from build123d import *

# Parameters (mm, degrees)
SKETCH1_R                         = 4.9276
BOSS_EXTRUDE1_DEPTH               = 7.9375
SKETCH4_R                         = 4.9276
BOSS_EXTRUDE2_DEPTH               = 3.175
BOSS_EXTRUDE2_TAPER               = 45
F_1_4_20_TAPPED_HOLE1_D           = 5.1054
F_1_4_20_TAPPED_HOLE1_DEPTH       = 16.51
F_1_4_20_TAPPED_HOLE1_CSINK_D     = 8.9154
F_1_4_20_TAPPED_HOLE1_CSINK_ANGLE = 90
F_1_4_20_TAPPED_HOLE1_TIP         = 1.533816902


with BuildPart() as part:
    # Sketch1 → Boss-Extrude1 (new body)
    with BuildSketch(Plane.XY):
        with Locations((-11.193990041, 3.085910768)):
            Circle(SKETCH1_R)
    extrude(amount=BOSS_EXTRUDE1_DEPTH)

    # Sketch4 → Boss-Extrude2 (add)
    with BuildSketch(Plane(origin=(0, 0, 0), x_dir=(-1, 0, 0), z_dir=(0, 0, -1))):
        with Locations((11.193990041, 3.085910768)):
            Circle(SKETCH4_R)
    extrude(amount=BOSS_EXTRUDE2_DEPTH, taper=BOSS_EXTRUDE2_TAPER)

    # 1/4-20 Tapped Hole1
    with Locations(Plane.XY.offset(7.9375)):
        with Locations((-11.193990041, 3.085910768)):
            CounterSinkHole(F_1_4_20_TAPPED_HOLE1_D / 2, F_1_4_20_TAPPED_HOLE1_CSINK_D / 2, depth=F_1_4_20_TAPPED_HOLE1_DEPTH, counter_sink_angle=F_1_4_20_TAPPED_HOLE1_CSINK_ANGLE)
            with Locations((0, 0, -(F_1_4_20_TAPPED_HOLE1_DEPTH + F_1_4_20_TAPPED_HOLE1_TIP / 2))):  # 118° drill point
                Cone(0, F_1_4_20_TAPPED_HOLE1_D / 2, F_1_4_20_TAPPED_HOLE1_TIP, mode=Mode.SUBTRACT)


solid = part.part
Build history of the part. All positions in model axes, mm. Round coordinates to 2 decimals unless told otherwise and drop trailing zeros. Write each loop counter-clockwise with the first axis right and the second up, starting at its lowest first coordinate (ties: lowest second). Pieces come first, ordered by that corner, then holes. Notation, with made-up numbers: M 73.25,-29 L 95.25,-29 A15 cw 95.25,-13 Z; hole C -7.5,-2.75 d3. An arc over 180 degrees is marked long. Answer as a JSON object with one key per item and string values. Group by question number.
(1) Mould opens along Y. For faces 1 (the cylindrical face through (-8.644, 3.198, 1.77)), 2 (the cylindrical face through (-6.494, 4.566, 3.913)) say: pulls with the +Y half, pulls with the -Y half, needs draft (parallel to the pull), parting line crosses it, or undercut.
(2) Cut at A-A (z = 0.75). Give the cut face in (x, y), and give its area (3 significant figures).
(3) Drill centre lines: L1, parallel to Y at x = -11.25, z = 4.5; L2, parallel to X at y = 0.75, z = 5.75; L3, parallel to X at y = 4.5, z = 1.75. Where is each one in solid material? Low to high.
(4) Flat gauge pins, fed straight in: pin 1 (1.5 mm diameter, centred on y = 0, z = 1.5, fed in from +X); pin 2 (2 mm diameter, centred on y = 1.5, z = 0.5, fed in from -X); pin 3 (2 mm diameter, centred on y = 5.5, z = -1, fed in from +X). Where does each tip first touch, or does it go through?
(5) Cut at B-B (z = 6.25). Give the cut face in (x, y).
Responses:
{
 "1": {"face 1": "undercut", "face 2": "parting line crosses it"},
 "2": {"outline": "C -11.19,3.09 d9.86; hole C -11.19,3.09 d5.11", "area": "55.8 mm2"},
 "3": {"L1": "y = -1.84 to 0.53, 5.64 to 8.01", "L2": "x = -15.53 to -12.22, -10.16 to -6.86", "L3": "x = -15.91 to -13.32, -9.07 to -6.47"},
 "4": {"pin 1": "stops at x = -6.86", "pin 2": "stops at x = -16.09", "pin 3": "stops at x = -6.79"},
 "5": {"outline": "C -11.19,3.09 d9.86; hole C -11.19,3.09 d5.54"}
}
